Design review of the part built by this model. Coordinates are the model's own, in mm. A direction names the side the tool comes from. Give positions to 0.01 mm unless a question says otherwise; leave off trailing zeros. Order: outer loops, then holes, each group sorted by start corner. A loop starts at its lowest first (then second) coordinate and runs counter-clockwise, first axis right, second up.
```python
from build123d import *

# Parameters (mm, degrees)
SKETCH_1_W          = 30
SKETCH_1_H          = 38
EXTRUDE_1_DEPTH     = 12
CUT_EXTRUDE_START   = 3
SKETCH_1_4_W        = 26
SKETCH_1_4_H        = 26
CUT_EXTRUDE_1_DEPTH = 14
SKETCH_1_6_W        = 16.5
SKETCH_1_6_H        = 26
CUT_EXTRUDE_2_DEPTH = 2
SKETCH_1_7_R        = 1.25
CUT_EXTRUDE_5_DEPTH = 21
SKETCH_1_8_R        = 2.25
CUT_EXTRUDE_6_DEPTH = 5
SKETCH_3_W          = 13
SKETCH_3_H          = 7
CUT_EXTRUDE_7_DEPTH = 7
FILLET_1_R          = 1
FILLET_2_R          = 1


with BuildPart() as part:
    # 草图1 → 凸台-拉伸1 (new body)
    with BuildSketch(Plane(origin=(0, 0, 0), x_dir=(1, 0, 0), z_dir=(0, 1, 0))):
        Rectangle(SKETCH_1_W, SKETCH_1_H)
    extrude(amount=EXTRUDE_1_DEPTH)

    # 草图1<4> → 切除-拉伸1 (cut)
    with BuildSketch(Plane(origin=(0, 0, 0), x_dir=(1, 0, 0), z_dir=(0, 1, 0)).offset(CUT_EXTRUDE_START)):
        Rectangle(SKETCH_1_4_W, SKETCH_1_4_H)
    extrude(amount=CUT_EXTRUDE_1_DEPTH, mode=Mode.SUBTRACT)

    # 草图1<6> → 切除-拉伸2 (cut)
    with BuildSketch(Plane(origin=(0, 0, 0), x_dir=(1, 0, 0), z_dir=(0, 1, 0)).offset(CUT_EXTRUDE_START)):
        Rectangle(SKETCH_1_6_W, SKETCH_1_6_H)
    extrude(amount=-CUT_EXTRUDE_2_DEPTH, mode=Mode.SUBTRACT)

    # 草图1<7> → 切除-拉伸5 (cut)
    with BuildSketch(Plane(origin=(0, 0, 0), x_dir=(1, 0, 0), z_dir=(0, 1, 0))):
        with Locations(Location((-11.3, 16, 0), (0, 0, 90))):
            Circle(SKETCH_1_7_R)
        with Locations(Location((11.3, 16, 0), (0, 0, 90))):
            Circle(SKETCH_1_7_R)
        with Locations(Location((11.3, -16, 0), (0, 0, 90))):
            Circle(SKETCH_1_7_R)
        with Locations(Location((-11.3, -16, 0), (0, 0, 90))):
            Circle(SKETCH_1_7_R)
    extrude(amount=CUT_EXTRUDE_5_DEPTH, mode=Mode.SUBTRACT)

    # 草图1<8> → 切除-拉伸6 (cut)
    with BuildSketch(Plane(origin=(0, 0, 0), x_dir=(1, 0, 0), z_dir=(0, 1, 0))):
        with Locations(Location((-11.3, 16, 0), (0, 0, 270))):
            Circle(SKETCH_1_8_R)
        with Locations(Location((11.3, 16, 0), (0, 0, 90))):
            Circle(SKETCH_1_8_R)
        with Locations(Location((11.3, -16, 0), (0, 0, 270))):
            Circle(SKETCH_1_8_R)
        with Locations(Location((-11.3, -16, 0), (0, 0, 90))):
            Circle(SKETCH_1_8_R)
    extrude(amount=CUT_EXTRUDE_6_DEPTH, mode=Mode.SUBTRACT)

    # 草图3 → 切除-拉伸7 (cut)
    with BuildSketch(Plane.XY.offset(-19)):
        with Locations((0, 6.5)):
            Rectangle(SKETCH_3_W, SKETCH_3_H)
    extrude(amount=CUT_EXTRUDE_7_DEPTH, mode=Mode.SUBTRACT)

    # 圆角1
    fillet_1_edges = [part.edges().sort_by_distance(p)[0] for p in [
        (6.5, 3, -16),
        (6.5, 10, -16),
        (-6.5, 10, -16),
        (-6.5, 3, -16),
    ]]
    fillet(fillet_1_edges, radius=FILLET_1_R)

    # 圆角2
    fillet_2_edges = [part.edges().sort_by_distance(p)[0] for p in [
        (0, 3, -19),
        (6.5, 6.5, -19),
        (0, 10, -19),
        (-6.5, 6.5, -19),
        (6.207106781, 3.292893219, -19),
        (6.207106781, 9.707106781, -19),
        (-6.207106781, 9.707106781, -19),
        (-6.207106781, 3.292893219, -19),
    ]]
    fillet(fillet_2_edges, radius=FILLET_2_R)


solid = part.part
```
1. Take a section at D-D (x = -11.3). State the section outline as (y, z) points, then the cut area to 3 significant figures.
Recorded:
outline: (0, -19) - (12, -19) - (12, -17.25) - (5, -17.25) - (5, -18.25) - (0, -18.25) - close; (0, -13.75) - (5, -13.75) - (5, -14.75) - (12, -14.75) - (12, -13) - (3, -13) - (3, 13) - (12, 13) - (12, 14.75) - (5, 14.75) - (5, 13.75) - (0, 13.75) - close; (0, 18.25) - (5, 18.25) - (5, 17.25) - (12, 17.25) - (12, 19) - (0, 19) - close
area: 142 mm2
2. Take a section at C-C (y = 6.75). State the section outline as (x, z) points.
Recorded:
outline: (-15, -19) - (-7.5, -19) arc R1 ccw to (-6.5, -18) - (-6.5, -13) - (-13, -13) - (-13, 13) - (13, 13) - (13, -13) - (6.5, -13) - (6.5, -18) arc R1 ccw to (7.5, -19) - (15, -19) - (15, 19) - (-15, 19) - close; hole circle Ø2.5 at (-11.3, -16); hole circle Ø2.5 at (-11.3, 16); hole circle Ø2.5 at (11.3, -16); hole circle Ø2.5 at (11.3, 16)
3. For line 1 along X through (y, z) = (7.5, 16); line 2 along X through (y, z) = (1.6, -16); line 3 along X through (y, z) = (7.75, 6), list the stretches that pass through material, from the lowest coordinate up.
Recorded:
line 1: x = -15 to -12.55, -10.05 to 10.05, 12.55 to 15
line 2: x = -15 to -13.55, -9.05 to 9.05, 13.55 to 15
line 3: x = -15 to -13, 13 to 15
4. Draft analysis for pull direction X (two halves, no side actions). For faces 6 (the face through (-14, 12, 0)), 7 (the face through (-15, 6, 0)), 8 (the face through (0, 1, 0)), state which applies: pulls with the +X half, pulls with the -X half, needs draft (parallel to the pull), parting line crosses it, or undercut.
Recorded:
face 6: needs draft
face 7: pulls with the -X half
face 8: undercut
5. Take a section at B-B (z = -16). State the section outline as (x, y) points.
Recorded:
outline: (-15, 0) - (-13.55, 0) - (-13.55, 5) - (-12.55, 5) - (-12.55, 12) - (-15, 12) - close; (-10.05, 5) - (-9.05, 5) - (-9.05, 0) - (9.05, 0) - (9.05, 5) - (10.05, 5) - (10.05, 12) - (-10.05, 12) - close; (12.55, 5) - (13.55, 5) - (13.55, 0) - (15, 0) - (15, 12) - (12.55, 12) - close; hole (-6.5, 4) arc R1 ccw to (-5.5, 3) - (5.5, 3) arc R1 ccw to (6.5, 4) - (6.5, 9) arc R1 ccw to (5.5, 10) - (-5.5, 10) arc R1 ccw to (-6.5, 9) - close
6. Machinability: for faces 1 (the face through (0, 10, -16)), 2 (the face through (0, 6, 19)), 3 (the face through (-11.976, 2.465, 13.854)), 4 (the face through (0, 11, -13)), 5 (the face through (10.06, 8.45, -15.84)), which of the approach directions +Z, -Z, +X, -X, +Y, -Y give a long, thin tool a straight path to every point of the face, cutting with its end or side? Answer none if there is none.
Recorded:
face 1: -Z
face 2: +Z, +X, -X, +Y, -Y
face 3: -Y
face 4: +Y
face 5: +Y, -Y
7. For pin 1 (13 mm diameter, centred on x = -4, z = 1.5, fed in from +Y); pin 2 (4 mm diameter, centred on x = -3, z = -1.5, fed in from +Y), all flat-tipped, find the tip position at first contact; note any pin that passes through.
Recorded:
pin 1: stops at y = 3
pin 2: stops at y = 1
8. Take a section at A-A (x = -3.75). State the section outline as (y, z) points, then the cut area to 3 significant figures.
Recorded:
outline: (0, -19) - (2, -19) arc R1 ccw to (3, -18) - (3, -13) - (1, -13) - (1, 13) - (12, 13) - (12, 19) - (0, 19) - close; (10, -18) arc R1 ccw to (11, -19) - (12, -19) - (12, -13) - (10, -13) - close
area: 128 mm2
